For this review, take the finished solid that the model builds, in its own axes (mm). Face numbers are marked on the shaded views. Round coordinates to 2 decimals unless told otherwise and drop trailing zeros. One line per question, with ' | ' between items. Start each with the question number.
1) We need section A-A (y = -0.25). State how many separate pieces and enclosed holes the cut face has, and give its area (3 significant figures).
2) For probe 1 along X at (y, z) = (1.5, -0.05); probe 2 along X at (y, z) = (1, 0.05); probe 3 along Y at (x, z) = (0, 0.1), list the stretches that pass through material, from the lowest coordinate up. Write a range as from..to.
3) Mouldability with a two-part tool opening along Z and no side actions: class the marked faces 1, 2, 3 and 4 as pulls with the +Z half, pulls with the -Z half, needs draft (parallel to the pull), parting line crosses it, or undercut.
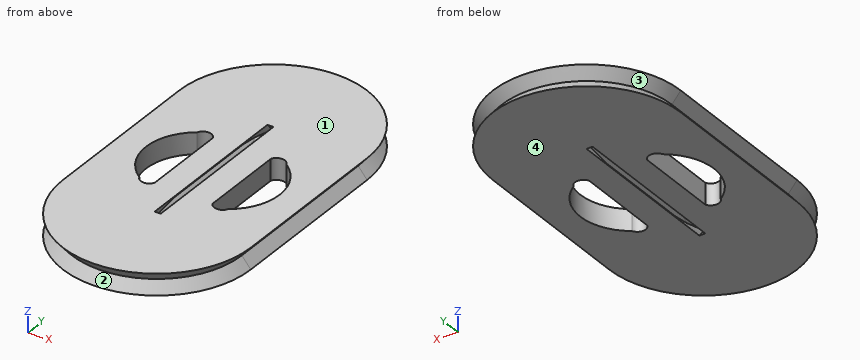
```python
from build123d import *

# Parameters (mm, degrees)
PAD_DEPTH    = 0.25
PAD_TAPER    = -40
POCKET_DEPTH = 1


with BuildPart() as part:
    # Sketch → Pad (new body, symmetric)
    with BuildSketch(Plane.XY):
        with BuildLine():
            ThreePointArc((2, 2.538372), (0, 4.538372), (-2, 2.538372))
            Line((-2, 2.538372), (-2, -1.461628))
            ThreePointArc((-2, -1.461628), (0, -3.461628), (2, -1.461628))
            Line((2, -1.461628), (2, 2.538372))
        make_face()
        with BuildLine():
            ThreePointArc((-0.135939, 2.669636), (-0.245341, 2.62432), (-0.290657, 2.514917))
            Line((-0.290657, -1.471332), (-0.290657, 2.514917))
            ThreePointArc((-0.290657, -1.471332), (-0.245341, -1.580734), (-0.135939, -1.62605))
            Line((0.114686, -1.62605), (-0.135939, -1.62605))
            ThreePointArc((0.114686, -1.62605), (0.224088, -1.580734), (0.269404, -1.471332))
            Line((0.269404, 2.514917), (0.269404, -1.471332))
            ThreePointArc((0.269404, 2.514917), (0.224088, 2.62432), (0.114686, 2.669636))
            Line((-0.135939, 2.669636), (0.114686, 2.669636))
        make_face(mode=Mode.SUBTRACT)
    extrude(amount=PAD_DEPTH, both=True, taper=PAD_TAPER)

    # Sketch001 (on Face20 of Pad) → Pocket (cut)
    with BuildSketch(Plane.XY.offset(0.25)):
        with BuildLine():
            Line((-0.681278, 1.458789), (-0.681278, -0.541211))
            ThreePointArc((-1.044875, -0.537362), (-0.864311, -0.655939), (-0.681278, -0.541211))
            ThreePointArc((-1.051415, 1.46106), (-1.572153, 0.460134), (-1.044875, -0.537362))
            ThreePointArc((-0.681278, 1.458789), (-0.865584, 1.584104), (-1.051415, 1.46106))
        make_face()
        with BuildLine():
            Line((0.681278, 1.458789), (0.681278, -0.541211))
            ThreePointArc((0.681278, -0.541211), (0.864311, -0.655939), (1.044875, -0.537362))
            ThreePointArc((1.044875, -0.537362), (1.572153, 0.460134), (1.051415, 1.46106))
            ThreePointArc((1.051415, 1.46106), (0.865584, 1.584104), (0.681278, 1.458789))
        make_face()
    extrude(amount=-POCKET_DEPTH, mode=Mode.SUBTRACT)


solid = part.part
```
Answers below:
1) separate pieces: 4 | enclosed holes: 0 | area: 1.27 mm^2
2) probe 1: -2.04..-1.03, -0.7..-0.25, 0.23..0.7, 1.03..2.04 | probe 2: -2.04..-1.45, -0.68..-0.25, 0.23..0.68, 1.45..2.04 | probe 3: -3.55..-1.54, 2.59..4.62
3) face 1: pulls with the +Z half | face 2: undercut | face 3: undercut | face 4: pulls with the -Z half
